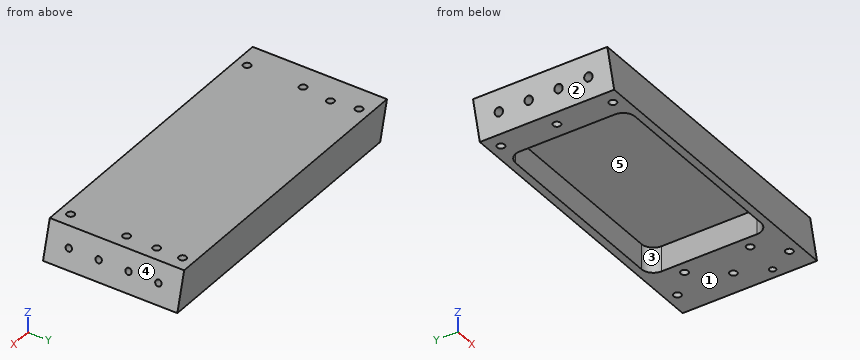
```python
from build123d import *

# Parameters (mm, degrees)
F1_DEPTH  = 90
F3_DEPTH  = 17
F5_D      = 5.5
F5_DEPTH  = 17.4
F5_TIP    = 1.6523667023
F7_D      = 5
F9_D      = 5
F9_DEPTH  = 10
F9_TIP    = 1.5021515476
F11_D     = 4.2
F11_DEPTH = 17.4
F11_TIP   = 1.2618073
F13_D     = 4.2
F13_DEPTH = 13.4
F13_TIP   = 1.2618073
F15_D     = 5
F15_DEPTH = 18
F15_TIP   = 1.5021515476


with BuildPart() as f1:
    # F0 (on Front) → F1 (new body)
    with BuildSketch(Plane.XZ):
        Polygon((200, 0), (0, 0), (6.72552473, -25.1), (206.72552473, -25.1), align=None)
    extrude(amount=F1_DEPTH)

    # F2 (on face) → F3 (cut)
    with BuildSketch(Plane(origin=(0, 0, -25.1), x_dir=(1, 0, 0), z_dir=(0, 0, -1))):
        with BuildLine():
            Line((158.72552473, 85), (106.72552473, 85))
            Line((106.72552473, 85), (34.72552473, 85))
            ThreePointArc((34.72552473, 85), (29.0686704805, 82.6568542495), (26.72552473, 77))
            Line((26.72552473, 77), (26.72552473, 13))
            ThreePointArc((26.72552473, 13), (29.0686704805, 7.3431457505), (34.72552473, 5))
            Line((34.72552473, 5), (158.72552473, 5))
            ThreePointArc((158.72552473, 5), (164.3823789795, 7.3431457505), (166.72552473, 13))
            Line((166.72552473, 13), (166.72552473, 77))
            ThreePointArc((166.72552473, 77), (164.3823789795, 82.6568542495), (158.72552473, 85))
        make_face()
    extrude(amount=-F3_DEPTH, mode=Mode.SUBTRACT)

    # F5
    with Locations(Plane(origin=(0, 0, 0), x_dir=(0, -1, 0), z_dir=(-0.9659258263, 0, -0.2588190451))):
        with Locations((15, -12.9927160641), (35, -12.9927160641), (55, -12.9927160641), (75, -12.9927160641)):
            Hole(F5_D / 2, depth=F5_DEPTH)
            with Locations((0, 0, -(F5_DEPTH + F5_TIP / 2))):  # 118° drill point
                Cone(0, F5_D / 2, F5_TIP, mode=Mode.SUBTRACT)

    # F7 (through all)
    with Locations(Plane.XY):
        with Locations((16.5, -7.5), (16.5, -45), (16.5, -82.5), (190.5, -82.5), (190.5, -45), (190.5, -7.5)):
            Hole(F7_D / 2)

    # F9
    with Locations(Plane.XY):
        with Locations((19, -25), (190.7, -24.7)):
            Hole(F9_D / 2, depth=F9_DEPTH)
            with Locations((0, 0, -(F9_DEPTH + F9_TIP / 2))):  # 118° drill point
                Cone(0, F9_D / 2, F9_TIP, mode=Mode.SUBTRACT)

    # F11
    with Locations(Plane(origin=(186.6025403784, 0, 50), x_dir=(0, 1, 0), z_dir=(0.9659258263, 0, 0.2588190451))):
        with Locations((-15, -64.7565250847), (-35, -64.7565250847), (-55, -64.7565250847), (-75, -64.7565250847)):
            Hole(F11_D / 2, depth=F11_DEPTH)
            with Locations((0, 0, -(F11_DEPTH + F11_TIP / 2))):  # 118° drill point
                Cone(0, F11_D / 2, F11_TIP, mode=Mode.SUBTRACT)

    # F13
    with Locations(Plane(origin=(0, 0, -25.1), x_dir=(1, 0, 0), z_dir=(0, 0, -1))):
        with Locations((199.72552473, 65)):
            Hole(F13_D / 2, depth=F13_DEPTH)
            with Locations((0, 0, -(F13_DEPTH + F13_TIP / 2))):  # 118° drill point
                Cone(0, F13_D / 2, F13_TIP, mode=Mode.SUBTRACT)

    # F15
    with Locations(Plane(origin=(0, 0, -25.1), x_dir=(1, 0, 0), z_dir=(0, 0, -1))):
        with Locations((174.72552473, 67), (174.72552473, 23)):
            Hole(F15_D / 2, depth=F15_DEPTH)
            with Locations((0, 0, -(F15_DEPTH + F15_TIP / 2))):  # 118° drill point
                Cone(0, F15_D / 2, F15_TIP, mode=Mode.SUBTRACT)


solid = f1.part
```
Work out the finished part from the listing and answer in its coordinate system (mm). Face numbers are marked on the shaded views. A direction names the side the tool comes from. Coordinates: 2 decimals unless noted, no trailing zeros. Loops run counter-clockwise (first coordinate to the right, second up) from the corner with the lowest first, then second, coordinate; pieces in that order, holes last. Notation, with made-up numbers: (-3.5, 6) -> (32.5, 6) arc R18 ccw to (32.5, 29) -> close; hole circle Ø11 at (-29.5, 5.5). An arc over 180 degrees is marked (long way). Answer as CSV lines item,"result".
Q1. Find the intervals of material crossed by probe 1 along Y at (x, z) = (190.7, -2.5); probe 2 along Y at (x, z) = (16.5, -20); probe 3 along X at (y, z) = (-65, -17), in increasing order.
Findings:
probe 1,"y = -90 to -84.99, -80.01 to -47.49, -42.51 to -27.2, -22.2 to -9.99, -5.01 to 0"
probe 2,"y = -90 to -85, -80 to -47.5, -42.5 to -10, -5 to 0"
probe 3,"x = 4.56 to 26.73, 166.73 to 173.23, 176.23 to 197.63, 201.83 to 204.56"
Q2. A tool of negligible diameter and unlimited length cuts with its end or side. For the marked faces 4 and 5, from which of +Z, -Z, +X, -X, +Y, -Y can it reach the whole face along a straight path? Write none if from no direction.
Findings:
face 4,"+Z, +X, +Y, -Y"
face 5,"-Z"
Q3. The part is cut by section B-B on x = 57.5. Write down the section's boundary in (y, z).
Findings:
outline,"(-90, -25.1) -> (-85, -25.1) -> (-85, -8.1) -> (-5, -8.1) -> (-5, -25.1) -> (0, -25.1) -> (0, 0) -> (-90, 0) -> close"
Q4. The part is cut by section A-A on y = -7.5. Write down the section's boundary in (x, z) (3 decimals).
Findings:
outline,"(0, 0) -> (6.726, -25.1) -> (14, -25.1) -> (14, 0) -> close; (19, -25.1) -> (28.916, -25.1) -> (28.916, -8.1) -> (164.535, -8.1) -> (164.535, -25.1) -> (188, -25.1) -> (188, 0) -> (19, 0) -> close; (193, -25.1) -> (206.726, -25.1) -> (200, 0) -> (193, 0) -> close"
Q5. For a pull along X with two mould halves and no side action, classify the marked faces 1, 2 and 3 as +X half, -X half, draft (parallel to the pull), parting line (faces both ways), or undercut.
Findings:
face 1,"draft"
face 2,"-X half"
face 3,"undercut"
Q6. The part is cut by section D-D on x = 32. Write down the section's boundary in (y, z), and give its area (3 significant figures).
Findings:
outline,"(-90, -25.1) -> (-84.52, -25.1) -> (-84.52, -8.1) -> (-5.48, -8.1) -> (-5.48, -25.1) -> (0, -25.1) -> (0, 0) -> (-90, 0) -> close"
area,"915 mm²"
Q7. Each of these flat-tipped pins is pushed along its axis until it touches: pin 1 (24 mm diameter, centred on x = 109, y = -33.5, fed in from -Z); pin 2 (4 mm diameter, centred on x = 190.5, y = -45, fed in from -Z); pin 3 (4.5 mm diameter, centred on x = 190.7, y = -24.7, fed in from +Z); pin 4 (5 mm diameter, centred on y = -69.5, z = -18.5, fed in from +X). Where does it stop, or does it pass through?
Findings:
pin 1,"stops at z = -8.1"
pin 2,"passes through"
pin 3,"stops at z = -10.15"
pin 4,"stops at x = 205.63"
Q8. The part is cut by section C-C on z = -21.25. State how many separate pieces and enclosed holes the cut face has, and give its area (3 significant figures).
Findings:
separate pieces,"1"
enclosed holes,"10"
area,"6,680 mm²"
